from build123d import *

# Parameters (mm, degrees)
SKETCH2_W           = 37.465
SKETCH2_H           = 24.13
BOSS_EXTRUDE1_DEPTH = 24.892
CUT_EXTRUDE1_DEPTH  = 20.701
CUT_EXTRUDE3_DEPTH  = 4.191
FILLET1_R           = 5.08
BOSS_EXTRUDE3_START = 2.286
BOSS_EXTRUDE3_DEPTH = 2.286
SKETCH8_R           = 1.905
CUT_EXTRUDE4_DEPTH  = 7.62


with BuildPart() as part:
    # Sketch2 → Boss-Extrude1 (new body)
    with BuildSketch(Plane.XY):
        with Locations((18.7325, 12.065)):
            Rectangle(SKETCH2_W, SKETCH2_H)
    extrude(amount=BOSS_EXTRUDE1_DEPTH)

    # Sketch3 → Cut-Extrude1 (cut)
    with BuildSketch(Plane.XY.offset(24.892)):
        with BuildLine():
            ThreePointArc((3.175, 16.637), (4.439712919, 19.690287081), (7.493, 20.955))
            Line((7.493, 20.955), (29.972, 20.955))
            ThreePointArc((29.972, 20.955), (33.025287081, 19.690287081), (34.29, 16.637))
            Line((34.29, 16.637), (34.29, 7.493))
            ThreePointArc((34.29, 7.493), (33.025287081, 4.439712919), (29.972, 3.175))
            Line((29.972, 3.175), (7.493, 3.175))
            ThreePointArc((7.493, 3.175), (4.439712919, 4.439712919), (3.175, 7.493))
            Line((3.175, 7.493), (3.175, 16.637))
        make_face()
    extrude(amount=-CUT_EXTRUDE1_DEPTH, mode=Mode.SUBTRACT)

    # Sketch4 → Cut-Extrude3 (cut)
    with BuildSketch(Plane.XY.offset(4.191)):
        with BuildLine():
            Line((32.086974483, 8.570131), (32.07077796, 10.882539488))
            add(Edge.make_bspline(
                [(32.07077796, 10.882539488), (32.073215089, 11.03512727), (32.05346317, 11.384531492), (31.98348624, 11.89897185), (31.690265244, 12.891461502), (30.781603575, 14.240804474), (29.41900903, 15.119220909), (28.414706523, 15.393168176), (27.909381539, 15.452204781), (27.554769457, 15.464756938), (27.429691001, 15.46229384)],
                knots=[0, 0, 0, 0.046875, 0.09375, 0.1875, 0.375, 0.625, 0.8125, 0.90625, 0.953125, 1, 1, 1], degree=2))
            Line((27.429691001, 15.46229384), (21.587714207, 15.44582783))
            add(Edge.make_bspline(
                [(21.587714207, 15.44582783), (21.462803996, 15.448731855), (21.106730304, 15.437338634), (20.595765352, 15.378996632), (19.591692577, 15.107051395), (18.225687665, 14.229774678), (17.316214622, 12.885953496), (17.020022679, 11.889285009), (16.949885556, 11.382167163), (16.92906595, 11.034797324), (16.930958193, 10.882006896)],
                knots=[0, 0, 0, 0.046875, 0.09375, 0.1875, 0.375, 0.625, 0.8125, 0.90625, 0.953125, 1, 1, 1], degree=2))
            Line((16.930958193, 10.882006896), (16.947147256, 8.570663591))
            add(Edge.make_bspline(
                [(16.947147256, 8.570663591), (16.944692803, 8.418076087), (16.96440505, 8.068669624), (17.034323571, 7.554221325), (17.32743188, 6.561698387), (18.235940341, 5.212252256), (19.598435143, 4.33368112), (20.60270654, 4.059619828), (21.108024818, 4.00052585), (21.462635472, 3.98793343), (21.587714207, 3.990382327)],
                knots=[0, 0, 0, 0.046875, 0.09375, 0.1875, 0.375, 0.625, 0.8125, 0.90625, 0.953125, 1, 1, 1], degree=2))
            Line((21.587714207, 3.990382327), (27.429691002, 4.006848338))
            add(Edge.make_bspline(
                [(27.429691002, 4.006848338), (27.554600877, 4.003929875), (27.910675883, 4.015281941), (28.421647575, 4.073564883), (29.425751775, 4.345394065), (30.791858076, 5.22251289), (31.701486436, 6.566228943), (31.997793574, 7.562863188), (32.067989311, 8.069972924), (32.088849066, 8.417340355), (32.086974483, 8.570131)],
                knots=[0, 0, 0, 0.046875, 0.09375, 0.1875, 0.375, 0.625, 0.8125, 0.90625, 0.953125, 1, 1, 1], degree=2))
        make_face()
    extrude(amount=-CUT_EXTRUDE3_DEPTH, mode=Mode.SUBTRACT)

    # Fillet1
    fillet1_edges = [part.edges().sort_by_distance(p)[0] for p in [
        (0, 24.13, 12.446),
        (37.465, 24.13, 12.446),
        (37.465, 0, 12.446),
        (0, 0, 12.446),
    ]]
    fillet(fillet1_edges, radius=FILLET1_R)

    # Sketch7 → Boss-Extrude3 (add)
    with BuildSketch(Plane.XY.offset(24.892).offset(BOSS_EXTRUDE3_START)):
        with BuildLine():
            Line((6.44525, 1.2065), (31.01975, 1.2065))
            ThreePointArc((31.01975, 1.2065), (34.252642204, 2.545607796), (35.59175, 5.7785))
            Line((35.59175, 5.7785), (35.59175, 18.3515))
            ThreePointArc((35.59175, 18.3515), (34.252642204, 21.584392204), (31.01975, 22.9235))
            Line((31.01975, 22.9235), (6.44525, 22.9235))
            ThreePointArc((6.44525, 22.9235), (3.212357796, 21.584392204), (1.87325, 18.3515))
            Line((1.87325, 18.3515), (1.87325, 5.7785))
            ThreePointArc((1.87325, 5.7785), (3.212357796, 2.545607796), (6.44525, 1.2065))
        make_face()
        with BuildLine():
            Line((7.493, 20.955), (29.972, 20.955))
            ThreePointArc((29.972, 20.955), (33.025287081, 19.690287081), (34.29, 16.637))
            Line((34.29, 16.637), (34.29, 7.493))
            ThreePointArc((34.29, 7.493), (33.025287081, 4.439712919), (29.972, 3.175))
            Line((29.972, 3.175), (7.493, 3.175))
            ThreePointArc((7.493, 3.175), (4.439712919, 4.439712919), (3.175, 7.493))
            Line((3.175, 7.493), (3.175, 16.637))
            ThreePointArc((3.175, 16.637), (4.439712919, 19.690287081), (7.493, 20.955))
        make_face(mode=Mode.SUBTRACT)
    extrude(amount=-BOSS_EXTRUDE3_DEPTH)

    # Sketch8 → Cut-Extrude4 (cut)
    with BuildSketch(Plane.ZY):
        with Locations((12.446, 12.065)):
            Circle(SKETCH8_R)
    extrude(amount=-CUT_EXTRUDE4_DEPTH, mode=Mode.SUBTRACT)


solid = part.part
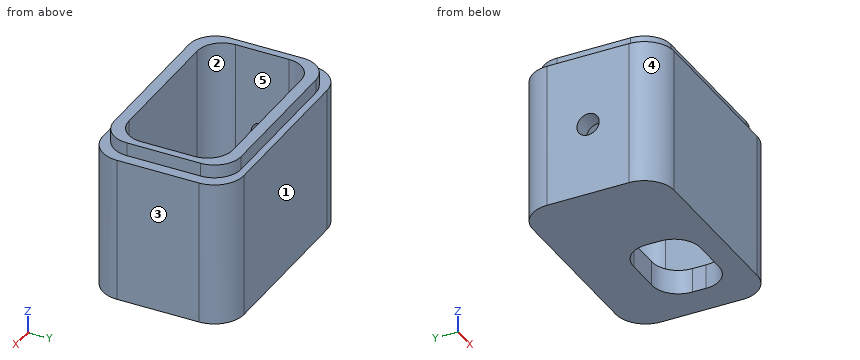
Read the model definition and answer for the solid it produces. Units are mm, in the model's axes. Face numbers are marked on the shaded views. A direction names the side the tool comes from. Round coordinates to 2 decimals unless told otherwise and drop trailing zeros. Write each loop counter-clockwise with the first axis right and the second up, starting at its lowest first coordinate (ties: lowest second). Pieces come first, ordered by that corner, then holes.
1. Determine the mould class of the marked faces 1, 2 and 3 for opening direction X: pulls with the +X half, pulls with the -X half, needs draft (parallel to the pull), parting line crosses it, or undercut.
2. The part is cut by section B-B, the plane x = 9.5. Determine the outline of the cut face in (y, z) (1 decimal).
3. Which of the six approach directions +Z, -Z, +X, -X, +Y, -Y give full straight-line access (tool end or side, diameter ignored) to the marked faces 4 and 5?
4. Given pin 1 Ø7 at (x, y) = (25, 16.5) entering from +Z; pin 2 Ø3.5 at (y, z) = (12.065, 12.446) entering from -X; pin 3 Ø1.1 at (y, z) = (11, 26) entering from +X, each flat-ended and moving along its own axis, determine where each tip first touches the part or whether it passes through.
5. The part is cut by section C-C, the plane x = 24. Determine the outline of the cut face in (y, z) (1 decimal).
6. Straight lines are drawn through the part: L1, parallel to Y at x = 26, z = 22.5 (3 decimals); L2, parallel to X at y = 10.75, z = 22.75 (3 decimals); L3, parallel to X at y = 9, z = 25.5 (3 decimals). For each, find the intervals that lie inside material, in ascending order.
7. The part is cut by section D-D, the plane z = 12.5. Determine the outline of the cut face in (x, y) (3 decimals).
8. The part is cut by section A-A, the plane z = 20.5. Determine the outline of the cut face in (x, y) (3 decimals).
Values:
1. face 1: needs draft
1. face 2: undercut
1. face 3: pulls with the +X half
2. outline: (0, 0) - (24.1, 0) - (24.1, 24.9) - (22.9, 24.9) - (22.9, 27.2) - (21, 27.2) - (21, 4.2) - (3.2, 4.2) - (3.2, 27.2) - (1.2, 27.2) - (1.2, 24.9) - (0, 24.9) - close
3. face 4: +Z, -Z, -X, -Y
3. face 5: +Z
4. pin 1: stops at z = 4.19
4. pin 2: stops at x = 34.29
4. pin 3: stops at x = 35.59
5. outline: (0, 0) - (4, 0) - (4, 4.2) - (3.2, 4.2) - (3.2, 27.2) - (1.2, 27.2) - (1.2, 24.9) - (0, 24.9) - close; (15.5, 0) - (24.1, 0) - (24.1, 24.9) - (22.9, 24.9) - (22.9, 27.2) - (21, 27.2) - (21, 4.2) - (15.5, 4.2) - close
6. L1: y = 0 to 3.175, 20.955 to 24.13
6. L2: x = 0 to 3.175, 34.29 to 37.465
6. L3: x = 1.873 to 3.175, 34.29 to 35.592
7. outline: (0, 5.08) arc R5.08 ccw to (5.08, 0) - (32.385, 0) arc R5.08 ccw to (37.465, 5.08) - (37.465, 19.05) arc R5.08 ccw to (32.385, 24.13) - (5.08, 24.13) arc R5.08 ccw to (0, 19.05) - (0, 13.969) - (3.175, 13.969) - (3.175, 16.637) arc R4.318 cw to (7.493, 20.955) - (29.972, 20.955) arc R4.318 cw to (34.29, 16.637) - (34.29, 7.493) arc R4.318 cw to (29.972, 3.175) - (7.493, 3.175) arc R4.318 cw to (3.175, 7.493) - (3.175, 10.161) - (0, 10.161) - close
8. outline: (0, 5.08) arc R5.08 ccw to (5.08, 0) - (32.385, 0) arc R5.08 ccw to (37.465, 5.08) - (37.465, 19.05) arc R5.08 ccw to (32.385, 24.13) - (5.08, 24.13) arc R5.08 ccw to (0, 19.05) - close; hole (3.175, 7.493) arc R4.318 ccw to (7.493, 3.175) - (29.972, 3.175) arc R4.318 ccw to (34.29, 7.493) - (34.29, 16.637) arc R4.318 ccw to (29.972, 20.955) - (7.493, 20.955) arc R4.318 ccw to (3.175, 16.637) - close
